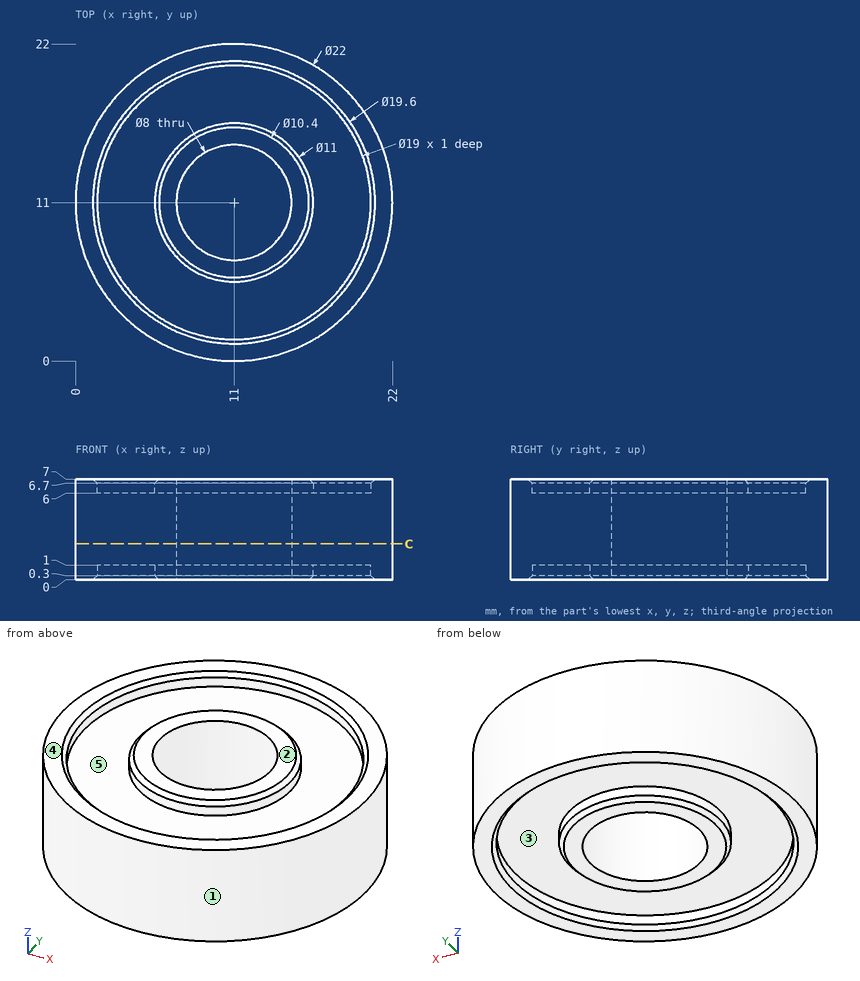
Check sheet for the drawn part. Datum: minimum x, y, z corner. Units: mm. A direction names the side the tool comes from. Coordinates: 2 decimals unless noted, no trailing zeros. Loops run counter-clockwise (first coordinate to the right, second up) from the corner with the lowest first, then second, coordinate; pieces in that order, holes last. Notation, with made-up numbers: (55.5, 41) -> (77.5, 41) arc R36 cw to (77.5, 76) -> close; hole circle Ø10 at (89, 35). An arc over 180 degrees is marked (long way). Write each question's results on one line, items separated by ' | '.
Item 1: Mould release check, pull along Y, two halves, no side actions. Record for the marked faces 1, 2 and 3: +Y half, -Y half, draft (parallel to the pull), parting line (faces both ways), or undercut.
Found:
face 1: parting line | face 2: draft | face 3: undercut
Item 2: Gauge pin test, flat ends, axial feed: pin 1 (1.5 mm diameter, centred on y = 19.5, z = 4, fed in from +X); pin 2 (3 mm diameter, centred on y = 19, z = 3.5, fed in from +X); pin 3 (4 mm diameter, centred on x = 3, z = 2, fed in from +Y). Record the tip position at first contact, or that the pin passes through.
Found:
pin 1: stops at x = 18.81 | pin 2: stops at x = 19.87 | pin 3: stops at y = 20.22
Item 3: Section check C-C, the plane z = 2.5. Enter the section's corners in (x, y), plus the area to 3 significant figures.
Found:
outline: circle Ø22 at (11, 11); hole circle Ø8 at (11, 11) | area: 330 mm2
Item 4: Material ranges on L1, parallel to Y at x = 11, z = 6.2; L2, parallel to Y at x = 11, z = 5.25; L3, parallel to Y at x = 13.5, z = 6.25, recorded low to high.
Found:
L1: y = 0 to 1.5, 5.5 to 7, 15 to 16.5, 20.5 to 22 | L2: y = 0 to 7, 15 to 22 | L3: y = 0.29 to 1.83, 6.1 to 7.88, 14.12 to 15.9, 20.17 to 21.71
Item 5: Tool access check on the marked faces 4 and 5. Record the directions out of +Z, -Z, +X, -X, +Y, -Y that give a thin tool (end or side, any length) a straight path to the whole face; none if there is none.
Found:
face 4: +Z, +X, -X, +Y, -Y | face 5: +Z
